from build123d import *

# Parameters (mm, degrees)
F0_W     = 70
F0_H     = 275
F1_DEPTH = 35
F2_W     = 17.5
F2_H     = 70
F3_DEPTH = 70.001
F5_DEPTH = 12.5
F6_DEPTH = 35.001


with BuildPart() as f1:
    # F0 (on Front) → F1 (new body)
    with BuildSketch(Plane.XZ):
        with Locations((35, 137.5)):
            Rectangle(F0_W, F0_H)
    extrude(amount=F1_DEPTH)

    # F2 (on face) → F3 (cut, through all)
    with BuildSketch(Plane.YZ.offset(70)):
        with Locations((-26.25, 240)):
            Rectangle(F2_W, F2_H)
    extrude(amount=-F3_DEPTH, mode=Mode.SUBTRACT)

    # F4 (on face) → F5 (cut, symmetric)
    with BuildSketch(Plane(origin=(0, 0, 0), x_dir=(-1, 0, 0), z_dir=(0, 1, 0))):
        Polygon((-70, 143.1957509073), (-70, 41.2869863212), (-35, 0), (0, 0), (0, 60.6217782649), align=None)
    extrude(amount=F5_DEPTH, both=True, mode=Mode.SUBTRACT)

    # F6 (cut, through all): a face of the model
    f6_faces = [f1.faces().sort_by_distance(p)[0] for p in [
        (58.3333333333, 0, 13.7623287737),
    ]]
    extrude(f6_faces, amount=-F6_DEPTH, mode=Mode.SUBTRACT)


solid = f1.part
Work out the finished part from the listing and answer in its coordinate system (mm). A direction names the side the tool comes from. Coordinates: 2 decimals unless noted, no trailing zeros. Loops run counter-clockwise (first coordinate to the right, second up) from the corner with the lowest first, then second, coordinate; pieces in that order, holes last. Notation, with made-up numbers: M 41.25,87 L 73.25,87 A29 ccw 73.25,125 Z; hole C 40,-33 d6. An arc over 180 degrees is marked long. Answer in a Markdown table with one row per item. Add a question column.
1. Find section B-B, the plane y = -30.5. Write down the section's boundary in (x, z), then the cut area to 3 significant figures.
2. Consider L1, parallel to Z at x = 24.5, y = -18; L2, parallel to Y at x = 28, z = 93; L3, parallel to Y at x = 21, z = 227.5. Determine where each line is inside the solid, lowest interval first.
3. A tool of negligible diameter and unlimited length cuts with its end or side. For faces 1 (the flat face through (35, -12.5, 57)), 2 (the flat face through (35, -26, 205)), 3 (the flat face through (35, -9, 275)), from which of +Z, -Z, +X, -X, +Y, -Y can it reach the whole face along a straight path? Write none if from no direction.
4. Find section D-D, the plane x = 64.5. Write down the section's boundary in (y, z), then the cut area to 3 significant figures.
5. Find section A-A, the plane x = 50.5. Write down the section's boundary in (y, z).
6. A flat-ended cylindrical pin translates along its axis: P1, Ø5, axis at x = 23, y = -28, coming from the +Z side. Find the tip coordinate at first contact, or state that the pin passes through.
7. Find section C-C, the plane z = 58. Write down the section's boundary in (x, y).
Reported:
| question | item | result |
|---|---|---|
| 1 | outline | M 0,0 L 35,0 L 70,41.29 L 70,205 L 0,205 Z |
| 1 | area | 13,600 mm^2 |
| 2 | L1 | z = 0 to 205 |
| 2 | L2 | y = -35 to -12.5 |
| 2 | L3 | y = -17.5 to 0 |
| 3 | face 1 | -Z, +X, +Y |
| 3 | face 2 | +Z, +X, -X, -Y |
| 3 | face 3 | +Z, +X, -X, +Y, -Y |
| 4 | outline | M -35,34.8 L -12.5,34.8 L -12.5,136.71 L 0,136.71 L 0,275 L -17.5,275 L -17.5,205 L -35,205 Z |
| 4 | area | 5,910 mm^2 |
| 5 | outline | M -35,18.28 L -12.5,18.28 L -12.5,120.19 L 0,120.19 L 0,275 L -17.5,275 L -17.5,205 L -35,205 Z |
| 6 | P1 | stops at z = 205 |
| 7 | outline | M 0,-35 L 70,-35 L 70,-12.5 L 0,-12.5 Z |
